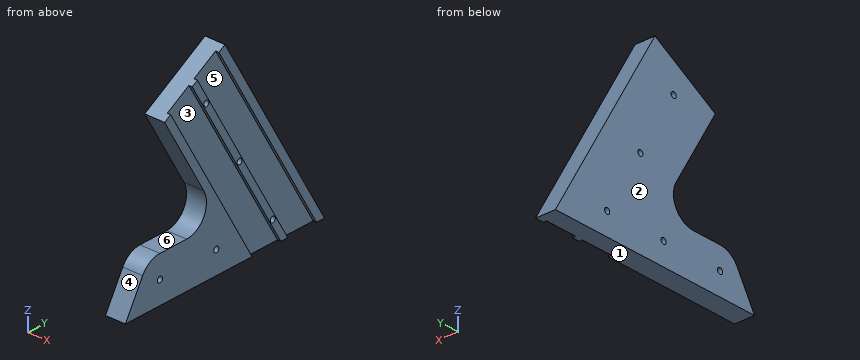
from build123d import *

# Parameters (mm, degrees)
PAD_DEPTH       = 18
SKETCH001_R     = 2.55
POCKET_DEPTH    = 18.001
SKETCH002_W     = 3
SKETCH002_H     = 25
POCKET002_DEPTH = 200.001


with BuildPart() as part:
    # Sketch → Pad (new body)
    with BuildSketch(Plane.YZ):
        with BuildLine():
            Line((0, 0), (200, 0))
            Line((200, 0), (100, 173.205081))
            Line((100, 173.205081), (39.378222, 138.205081))
            Line((39.378222, 138.205081), (78.756443, 70))
            ThreePointArc((61.435935, 40), (78.756443, 50), (78.756443, 70))
            Line((61.435935, 40), (34.641016, 40))
            ThreePointArc((34.641016, 40), (24.641016, 37.320508), (17.320508, 30))
            Line((17.320508, 30), (0, 0))
        make_face()
    extrude(amount=PAD_DEPTH)

    # Sketch001 (on Face10 of Pad) → Pocket (cut, through all)
    with BuildSketch(Plane.YZ.offset(18)):
        with Locations((81.236116, 135.705081)):
            Circle(SKETCH001_R)
        with Locations((114.637296, 77.85254)):
            Circle(SKETCH001_R)
        with Locations((148.038476, 20)):
            Circle(SKETCH001_R)
        with Locations((91.339746, 20)):
            Circle(SKETCH001_R)
        with Locations((34.641016, 20)):
            Circle(SKETCH001_R)
    extrude(amount=-POCKET_DEPTH, mode=Mode.SUBTRACT)

    # Sketch002 (on Face8 of Clone001) → Pocket002 (cut, through all)
    with BuildSketch(Plane(origin=(0, -50, 86.60254), x_dir=(1, 0, 0), z_dir=(0, -0.5, 0.866025))):
        with Locations((16.5, 153.705081)):
            Rectangle(SKETCH002_W, SKETCH002_H)
        with Locations((16.5, 122.705081)):
            Rectangle(SKETCH002_W, SKETCH002_H)
    extrude(amount=-POCKET002_DEPTH, mode=Mode.SUBTRACT)


solid = part.part
The listing builds one solid part. Answer for the finished solid, in the listing's coordinates (mm). Face numbers are marked on the shaded views. A direction names the side the tool comes from. Coordinates: 2 decimals unless noted, no trailing zeros. Write each loop counter-clockwise with the first axis right and the second up, starting at its lowest first coordinate (ties: lowest second). Pieces come first, ordered by that corner, then holes. Notation, with made-up numbers: M 89,-40 L 118,-40 A24 cw 118,-11 Z; hole C 33.25,20.5 d10. An arc over 180 degrees is marked long. Put each result on its own line as item: value. Start each with the question number.
1. Consider line 1 (Z direction, x = 13.5, y = 102); line 2 (X direction, y = 117, z = 115.5); line 3 (Y direction, x = 17, z = 75). Determine where each line is inside the solid, lowest interval first. Write a range as from..to.
2. Flat-ended cylindrical pins translate along their axes: P1, Ø3, axis at x = 12.5, z = 65, coming from the -Y side; P2, Ø3, axis at y = 114.64, z = 77.85, coming from the -X side; P3, Ø5.5, axis at x = 8.5, y = 42.5, coming from the +Z side; P4, Ø6, axis at x = 5, z = 93.5, coming from the +Y side. Find the tip coordinate at first contact, or state that the pin passes through.
3. A cutting plane is placed at B-B on y = 159. Write down the section's boundary in (x, z), then the cut area to 3 significant figures.
4. A cutting plane is placed at D-D on z = 55.5. Write down the section's boundary in (x, y), then the cut area to 3 significant figures.
5. A cutting plane is placed at C-C on x = 7.5. Write down the section's boundary in (y, z), then the cut area to 3 significant figures.
6. Which of the six approach directions +Z, -Z, +X, -X, +Y, -Y give full straight-line access (tool end or side, diameter ignored) to the marked faces 4, 5 and 6?
7. For a pull along Z with two mould halves and no side action, classify the marked faces 1, 2 and 3 as pulls with the +Z half, pulls with the -Z half, needs draft (parallel to the pull), parting line crosses it, or undercut.
8. A cutting plane is placed at A-A on z = 20. Write down the section's boundary in (x, y).
Resolved:
1. line 1: z = 0..169.74
1. line 2: x = 0..15
1. line 3: y = 75.87..83.95, 112.82..119.75, 148.62..156.7
2. P1: stops at y = 80.35
2. P2: passes through
2. P3: stops at z = 141.6
2. P4: stops at y = 147.75
3. outline: M 0,0 L 18,0 L 18,7.01 L 15,7.01 L 15,57.01 L 18,57.01 L 18,71.01 L 0,71.01 Z
3. area: 1,130 mm2
4. outline: M 0,80.92 L 18,80.92 L 18,95.21 L 15,95.21 L 15,124.08 L 18,124.08 L 18,131.01 L 15,131.01 L 15,159.87 L 18,159.87 L 18,167.96 L 0,167.96 Z
4. area: 1,390 mm2
5. outline: M 0,0 L 200,0 L 100,173.21 L 39.38,138.21 L 78.76,70 A20 cw 61.44,40 L 34.64,40 A20 ccw 17.32,30 Z; hole C 34.64,20 d5.1; hole C 81.24,135.71 d5.1; hole C 91.34,20 d5.1; hole C 114.64,77.85 d5.1; hole C 148.04,20 d5.1
5. area: 16,600 mm2
6. face 4: +Z, +X, -X, -Y
6. face 5: +X
6. face 6: +X, -X, -Y
7. face 1: pulls with the -Z half
7. face 2: needs draft
7. face 3: undercut
8. outline: M 0,11.55 L 18,11.55 L 18,32.09 L 0,32.09 Z; M 0,37.19 L 18,37.19 L 18,88.79 L 0,88.79 Z; M 0,93.89 L 18,93.89 L 18,115.71 L 15,115.71 L 15,144.57 L 18,144.57 L 18,145.49 L 0,145.49 Z; M 0,150.59 L 18,150.59 L 18,151.5 L 15,151.5 L 15,180.37 L 18,180.37 L 18,188.45 L 0,188.45 Z
